Can you work these out from the model? Positions are in its coordinate system, mm. Face numbers are marked on the shaded views. Coordinates: 2 decimals unless noted, no trailing zeros. Order: outer loops, then holes, each group sorted by start corner. A loop starts at its lowest first (then second) coordinate and runs counter-clockwise, first axis right, second up. Notation, with made-up numbers: (35, 67.25) -> (73, 67.25) arc R33 cw to (73, 96.25) -> close; hole circle Ø6 at (60.5, -8.5). An arc over 180 degrees is marked (long way). Answer as CSV lines item,"result".
from build123d import *

# Parameters (mm, degrees)
SKETCH1_R               = 40
SKETCH1_R_2             = 30
BOSS_EXTRUDE1_DEPTH     = 90
SKETCH2_R               = 7
CUT_EXTRUDE1_DEPTH      = 41
CUT_EXTRUDE1_DEPTH_BACK = 41


with BuildPart() as part:
    # Sketch1 → Boss-Extrude1 (new body, symmetric)
    with BuildSketch(Plane.XY):
        Circle(SKETCH1_R)
        Circle(SKETCH1_R_2, mode=Mode.SUBTRACT)
    extrude(amount=BOSS_EXTRUDE1_DEPTH, both=True)

    # Sketch2 → Cut-Extrude1 (cut, two sides)
    with BuildSketch(Plane(origin=(0, 0, 0), x_dir=(0, 0, -1), z_dir=(1, 0, 0))) as cut_extrude1_sk:
        with Locations((-72, 0)):
            Circle(SKETCH2_R)
        with Locations((72, 0)):
            Circle(SKETCH2_R)
    extrude(amount=CUT_EXTRUDE1_DEPTH, mode=Mode.SUBTRACT)
    extrude(cut_extrude1_sk.sketch, amount=-CUT_EXTRUDE1_DEPTH_BACK, mode=Mode.SUBTRACT)


solid = part.part
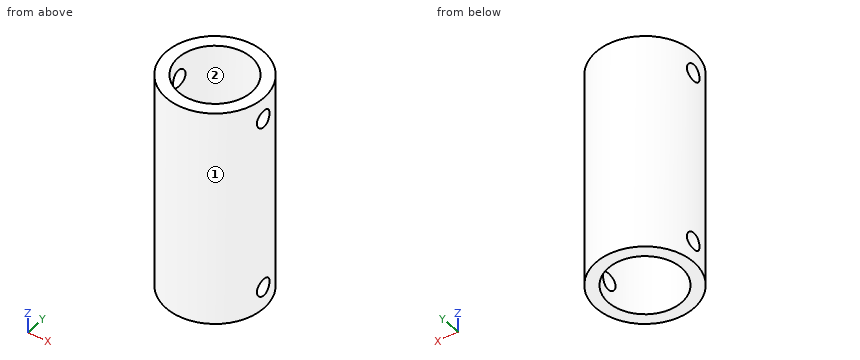
Q1. Imagine slicing it at B-B (y = 14). List the corners of the cut face in (x, z) for me.
Solution:
outline,"(-37.47, -90) -> (-26.53, -90) -> (-26.53, 90) -> (-37.47, 90) -> close; (26.53, -90) -> (37.47, -90) -> (37.47, 90) -> (26.53, 90) -> close"
Q2. Imagine slicing it at A-A (x = 0). List the corners of the cut face in (y, z) for me, and give its area (3 significant figures).
Solution:
outline,"(-40, -90) -> (-30, -90) -> (-30, 90) -> (-40, 90) -> close; (30, -90) -> (40, -90) -> (40, 90) -> (30, 90) -> close"
area,"3,600 mm2"
Q3. For P1, Ø4, axis at y = 0, z = 66.5, coming from the +X side; P2, Ø5, axis at x = 8.5, z = -39.5, coming from the -Y side; P3, Ø10, axis at x = -19, z = 39.5, coming from the +Y side; P4, Ø5, axis at x = 3, z = -17.5, coming from the -Y side, each with a flat end and sliding along its axis, tell me the tip position at first contact or that it passes through.
Solution:
P1,"x = 40"
P2,"y = -39.55"
P3,"y = 37.47"
P4,"y = -40"
Q4. Imagine slicing it at C-C (y = 0). List the corners of the cut face in (x, z) for me.
Solution:
outline,"(-40, -90) -> (-30, -90) -> (-30, -79) -> (-40, -79) -> close; (-40, -65) -> (-30, -65) -> (-30, 65) -> (-40, 65) -> close; (-40, 79) -> (-30, 79) -> (-30, 90) -> (-40, 90) -> close; (30, -90) -> (40, -90) -> (40, -79) -> (30, -79) -> close; (30, -65) -> (40, -65) -> (40, 65) -> (30, 65) -> close; (30, 79) -> (40, 79) -> (40, 90) -> (30, 90) -> close"
Q5. We'd pull the mould along X, two halves only. Please class the marked faces 1 and 2: pulls with the +X half, pulls with the -X half, needs draft (parallel to the pull), parting line crosses it, or undercut.
Solution:
face 1,"parting line crosses it"
face 2,"undercut"
Q6. Imagine slicing it at D-D (z = -47.5). List the corners of the cut face in (x, y) for me, and give its area (3 significant figures).
Solution:
outline,"circle Ø80 at (0, 0); hole circle Ø60 at (0, 0)"
area,"2,200 mm2"
Q7. If I drill on line 1 (Z direction, x = 37, y = 0); line 2 (Y direction, x = 0, z = 52); line 3 (X direction, y = 19, z = 11), over which ranges is the centre line in solid material (lowest first)?
Solution:
line 1,"-90 to -79, -65 to 65, 79 to 90"
line 2,"-40 to -30, 30 to 40"
line 3,"-35.2 to -23.22, 23.22 to 35.2"
